from build123d import *

# Parameters (mm, degrees)
SKETCH_1_W           = 100
SKETCH_1_H           = 70
EXTRUDE_1_DEPTH      = 10
SKETCH_6_W           = 5
SKETCH_6_H           = 5
CUT_EXTRUDE_4_DEPTH  = 5
SKETCH_7_W           = 5
SKETCH_7_H           = 5
CUT_EXTRUDE_5_DEPTH  = 3
SKETCH_8_R           = 1.05
CUT_EXTRUDE_6_DEPTH  = 42
SKETCH_10_W          = 100
SKETCH_10_H          = 70
CUT_EXTRUDE_7_DEPTH  = 3
SKETCH_11_W          = 7
SKETCH_11_H          = 70
CUT_EXTRUDE_8_DEPTH  = 5
SKETCH_12_W          = 7
SKETCH_12_H          = 70
CUT_EXTRUDE_9_DEPTH  = 5
SKETCH_15_W          = 82
SKETCH_15_H          = 52
CUT_EXTRUDE_12_DEPTH = 3
SKETCH_16_W          = 5
SKETCH_16_H          = 5
SKETCH_16_R          = 1.05
EXTRUDE_2_DEPTH      = 5
SKETCH_18_W          = 80
SKETCH_18_H          = 3
CUT_EXTRUDE_13_DEPTH = 10
SKETCH_19_W          = 82
SKETCH_19_H          = 52
CUT_EXTRUDE_14_DEPTH = 3
SKETCH_20_W          = 5
SKETCH_20_H          = 5
CUT_EXTRUDE_15_DEPTH = 3


with BuildPart() as part:
    # 草圖1 → 填料-伸長1 (new body)
    with BuildSketch(Plane.XY):
        with Locations((-39.08671555, 7.98136646)):
            Rectangle(SKETCH_1_W, SKETCH_1_H)
    extrude(amount=EXTRUDE_1_DEPTH)

    # 草圖6 → 除料-伸長4 (cut)
    with BuildSketch(Plane.XY.offset(10)):
        with Locations((3.41328445, 40.48136646)):
            Rectangle(SKETCH_6_W, SKETCH_6_H)
        with Locations((-81.58671555, 40.48136646)):
            Rectangle(SKETCH_6_W, SKETCH_6_H)
        with Locations((-81.58671555, -24.51863354)):
            Rectangle(SKETCH_6_W, SKETCH_6_H)
        with Locations((3.41328445, -24.51863354)):
            Rectangle(SKETCH_6_W, SKETCH_6_H)
    extrude(amount=-CUT_EXTRUDE_4_DEPTH, mode=Mode.SUBTRACT)

    # 草圖7 → 除料-伸長5 (cut)
    with BuildSketch(Plane(origin=(0, 0, 0), x_dir=(-1, 0, 0), z_dir=(0, 0, -1))):
        with Locations((81.58671555, 40.48136646)):
            Rectangle(SKETCH_7_W, SKETCH_7_H)
        with Locations((-3.41328445, 40.48136646)):
            Rectangle(SKETCH_7_W, SKETCH_7_H)
        with Locations((81.58671555, -24.51863354)):
            Rectangle(SKETCH_7_W, SKETCH_7_H)
        with Locations((-3.41328445, -24.51863354)):
            Rectangle(SKETCH_7_W, SKETCH_7_H)
    extrude(amount=-CUT_EXTRUDE_5_DEPTH, mode=Mode.SUBTRACT)

    # 草圖8 → 除料-伸長6 (cut)
    with BuildSketch(Plane(origin=(0, 0, 0), x_dir=(-1, 0, 0), z_dir=(0, 0, -1))):
        with Locations((-3.41328445, 40.48136646)):
            Circle(SKETCH_8_R)
        with Locations((81.58671555, 40.48136646)):
            Circle(SKETCH_8_R)
        with Locations((81.58671555, -24.51863354)):
            Circle(SKETCH_8_R)
        with Locations((-3.41328445, -24.51863354)):
            Circle(SKETCH_8_R)
    extrude(amount=-CUT_EXTRUDE_6_DEPTH, mode=Mode.SUBTRACT)

    # 草圖10 → 除料-伸長7 (cut)
    with BuildSketch(Plane.XY):
        with Locations((-39.08671555, 7.98136646)):
            Rectangle(SKETCH_10_W, SKETCH_10_H)
    extrude(amount=CUT_EXTRUDE_7_DEPTH, mode=Mode.SUBTRACT)

    # 草圖11 → 除料-伸長8 (cut)
    with BuildSketch(Plane(origin=(10.91328445, 0, 0), x_dir=(0, 0, -1), z_dir=(1, 0, 0))):
        with Locations((-6.5, 7.98136646)):
            Rectangle(SKETCH_11_W, SKETCH_11_H)
    extrude(amount=-CUT_EXTRUDE_8_DEPTH, mode=Mode.SUBTRACT)

    # 草圖12 → 除料-伸長9 (cut)
    with BuildSketch(Plane.ZY.offset(89.08671555)):
        with Locations((6.5, 7.98136646)):
            Rectangle(SKETCH_12_W, SKETCH_12_H)
    extrude(amount=-CUT_EXTRUDE_9_DEPTH, mode=Mode.SUBTRACT)

    # 草圖15 → 除料-伸長12 (cut)
    with BuildSketch(Plane.XY.offset(10)):
        with BuildLine():
            Line((-83.08671555, 34.98136646), (-83.08671555, -19.01863354))
            ThreePointArc((-83.08671555, -19.01863354), (-82.500929112, -20.432847103), (-81.08671555, -21.01863354))
            Line((-81.08671555, -21.01863354), (2.91328445, -21.01863354))
            ThreePointArc((2.91328445, -21.01863354), (4.327498013, -20.432847103), (4.91328445, -19.01863354))
            Line((4.91328445, -19.01863354), (4.91328445, 34.98136646))
            ThreePointArc((4.91328445, 34.98136646), (4.327498013, 36.395580022), (2.91328445, 36.98136646))
            Line((2.91328445, 36.98136646), (-81.08671555, 36.98136646))
            ThreePointArc((-81.08671555, 36.98136646), (-82.500929112, 36.395580022), (-83.08671555, 34.98136646))
        make_face()
        with Locations((-39.08671555, 7.98136646)):
            Rectangle(SKETCH_15_W, SKETCH_15_H, mode=Mode.SUBTRACT)
    extrude(amount=-CUT_EXTRUDE_12_DEPTH, mode=Mode.SUBTRACT)

    # 草圖16 → 填料-伸長2 (add)
    with BuildSketch(Plane.XY.offset(5)):
        with Locations((-81.58671555, 40.48136646)):
            Rectangle(SKETCH_16_W, SKETCH_16_H)
        with Locations((-81.58671555, 40.48136646)):
            Circle(SKETCH_16_R, mode=Mode.SUBTRACT)
        with Locations((3.41328445, 40.48136646)):
            Rectangle(SKETCH_16_W, SKETCH_16_H)
        with Locations((3.41328445, 40.48136646)):
            Circle(SKETCH_16_R, mode=Mode.SUBTRACT)
        with Locations((3.41328445, -24.51863354)):
            Rectangle(SKETCH_16_W, SKETCH_16_H)
        with Locations((3.41328445, -24.51863354)):
            Circle(SKETCH_16_R, mode=Mode.SUBTRACT)
        with Locations((-81.58671555, -24.51863354)):
            Rectangle(SKETCH_16_W, SKETCH_16_H)
        with Locations((-81.58671555, -24.51863354)):
            Circle(SKETCH_16_R, mode=Mode.SUBTRACT)
    extrude(amount=EXTRUDE_2_DEPTH)

    # 草圖18 → 除料-伸長13 (cut)
    with BuildSketch(Plane.XY.offset(10)):
        with Locations((-39.08671555, 41.48136646)):
            Rectangle(SKETCH_18_W, SKETCH_18_H)
        with Locations((-39.08671555, -25.51863354)):
            Rectangle(SKETCH_18_W, SKETCH_18_H)
    extrude(amount=-CUT_EXTRUDE_13_DEPTH, mode=Mode.SUBTRACT)

    # 草圖19 → 除料-伸長14 (cut)
    with BuildSketch(Plane.XY.offset(10)):
        with Locations((-39.08671555, 7.98136646)):
            Rectangle(SKETCH_19_W, SKETCH_19_H)
    extrude(amount=-CUT_EXTRUDE_14_DEPTH, mode=Mode.SUBTRACT)

    # 草圖20 → 除料-伸長15 (cut)
    with BuildSketch(Plane(origin=(0, 0, 3), x_dir=(-1, 0, 0), z_dir=(0, 0, -1))):
        with Locations((81.58671555, 40.48136646)):
            Rectangle(SKETCH_20_W, SKETCH_20_H)
        with Locations((-3.41328445, 40.48136646)):
            Rectangle(SKETCH_20_W, SKETCH_20_H)
        with Locations((81.58671555, -24.51863354)):
            Rectangle(SKETCH_20_W, SKETCH_20_H)
        with Locations((-3.41328445, -24.51863354)):
            Rectangle(SKETCH_20_W, SKETCH_20_H)
    extrude(amount=-CUT_EXTRUDE_15_DEPTH, mode=Mode.SUBTRACT)


solid = part.part
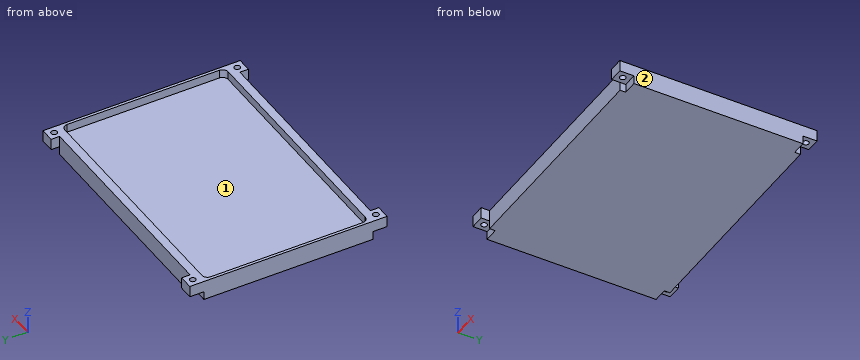
The listing builds one solid part. Answer for the finished solid, in the listing's coordinates (mm). Face numbers are marked on the shaded views. Round coordinates to 2 decimals unless told otherwise and drop trailing zeros. Loops run counter-clockwise (first coordinate to the right, second up) from the corner with the lowest first, then second, coordinate; pieces in that order, holes last. Notation, with made-up numbers: M 53,-17.5 L 75,-17.5 A11 cw 75,-5.5 Z; hole C -1,33 d2. An arc over 180 degrees is marked long. Write each question's results on one line, items separated by ' | '. Start each with the question number.
1) Find section B-B on z = 4.25. Write down the section's boundary in (x, y), plus the area to 3 significant figures.
2) Straight lines are drawn through the part: probe 1 along Y at (x, z) = (-61.5, 9); probe 2 along X at (y, z) = (32, 9.75); probe 3 along Y at (x, z) = (-49, 6.5). For each, find the intervals that lie inside material, in ascending order.
3) Find section C-C on y = 12. Write down the section's boundary in (x, z).
4) Find section A-A on x = -18. Write down the section's boundary in (y, z).
5) Each of these flat-tipped pins is pushed along its axis until it touches: pin 1 (1.5 mm diameter, centred on x = -37, z = 9, fed in from +Y); pin 2 (1.5 mm diameter, centred on x = -59.5, z = 4.5, fed in from -Y); pin 3 (1.6 mm diameter, centred on y = -22.5, z = 5, fed in from +X); pin 4 (8 mm diameter, centred on x = -7, y = -11, fed in from +Z). Where does it stop, or does it pass through?
6) Determine the mould class of the marked faces 1 and 2 for opening direction Y: pulls with the +Y half, pulls with the -Y half, needs draft (parallel to the pull), parting line crosses it, or undercut.
Final values:
1) outline: M -84.09,-22.02 L -79.09,-22.02 L -79.09,-24.02 L 0.91,-24.02 L 0.91,-22.02 L 5.91,-22.02 L 5.91,37.98 L 0.91,37.98 L 0.91,39.98 L -79.09,39.98 L -79.09,37.98 L -84.09,37.98 Z | area: 5,720 mm²
2) probe 1: -24.02 to -21.02, 36.98 to 39.98 | probe 2: -84.09 to -83.09, 4.91 to 5.91 | probe 3: -24.02 to 39.98
3) outline: M -84.09,3 L 5.91,3 L 5.91,10 L 4.91,10 L 4.91,7 L -83.09,7 L -83.09,10 L -84.09,10 Z
4) outline: M -24.02,3 L 39.98,3 L 39.98,10 L 36.98,10 L 36.98,7 L -21.02,7 L -21.02,10 L -24.02,10 Z
5) pin 1: y = 39.98 | pin 2: y = -24.02 | pin 3: x = 5.91 | pin 4: z = 7
6) face 1: undercut | face 2: needs draft
